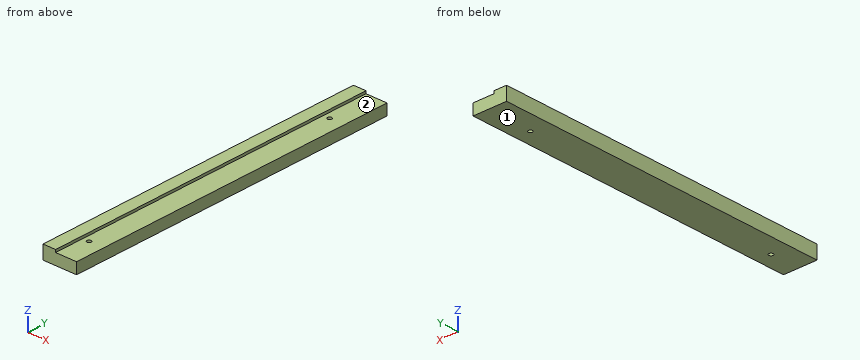
from build123d import *

# Parameters (mm, degrees)
SKETCH1_W         = 40
SKETCH1_H         = 400
EXTRUDE1_DEPTH    = 16
EXTRUDE2_REACH    = 402
SKETCH2_W         = 25
SKETCH2_H         = 3
M6_TAPPED_HOLE1_D = 5


with BuildPart() as part:
    # Sketch1 → Extrude1 (new body)
    with BuildSketch(Plane.XY):
        Rectangle(SKETCH1_W, SKETCH1_H)
    extrude(amount=EXTRUDE1_DEPTH)

    # Sketch2 → Extrude2 (cut, up to next)
    with BuildSketch(Plane.XZ.offset(200), mode=Mode.PRIVATE) as extrude2_sk1:
        with Locations((7.5, 14.5)):
            Rectangle(SKETCH2_W, SKETCH2_H)
    extrude2_tool1 = extrude(extrude2_sk1.sketch, amount=-EXTRUDE2_REACH, mode=Mode.PRIVATE) & part.part
    add(extrude2_tool1.solids().sort_by_distance((7.5, -200, 14.5))[0], mode=Mode.SUBTRACT)

    # M6 Tapped Hole1 (through all)
    with Locations(Plane(origin=(0, 0, 0), x_dir=(-1, 0, 0), z_dir=(0, 0, -1))):
        with Locations((-2.5, 145), (-2.5, -165)):
            Hole(M6_TAPPED_HOLE1_D / 2)


solid = part.part
Could you check a few things on this model? Use its own coordinates, in mm. Face numbers are marked on the shaded views. A direction names the side the tool comes from. Give positions to 0.01 mm unless a question says otherwise; leave off trailing zeros. Order: outer loops, then holes, each group sorted by start corner. A loop starts at its lowest first (then second) coordinate and runs counter-clockwise, first axis right, second up. Notation, with made-up numbers: (5, 41.5) - (39, 41.5) arc R22 ccw to (39, 62.5) - close; hole circle Ø4 at (61.25, 20.25). An arc over 180 degrees is marked (long way). Return JSON: item names as keys, results as strings. Group by question number.
Q1. Suppose I cut it at A-A, the plane y = 102. Please give me the cut outline in (x, z).
Q2. Which directions (+Z, -Z, +X, -X, +Y, -Y) give clear straight access to the entire face, cutting with the end or side of a thin tool? Please do the marked faces 1 and 2.
Q3. Will these pins go through, and if not, where does the flat tip stop? pin 1 Ø12.5 at (x, y) = (4.5, -36.5) entering from +Z; pin 2 Ø0.9 at (y, z) = (-2, 14.5) entering from +X.
Q4. Please list where these lines run through material, in increasing order: line 1 along Y through (x, z) = (2.5, 4.5); line 2 along X through (y, z) = (-165, 3); line 3 along Z through (x, y) = (13, 104.5). Write a range as [from, to].
Resolved:
{
 "1": {"outline": "(-20, 0) - (20, 0) - (20, 13) - (-5, 13) - (-5, 16) - (-20, 16) - close"},
 "2": {"face 1": "-Z, +X, -X, +Y, -Y", "face 2": "+Z, +X, +Y, -Y"},
 "3": {"pin 1": "stops at z = 13", "pin 2": "stops at x = -5"},
 "4": {"line 1": "y = [-200, -167.5], [-162.5, 142.5], [147.5, 200]", "line 2": "x = [-20, 0], [5, 20]", "line 3": "z = [0, 13]"}
}
